Part model, mm, in its own coordinate system. Face numbers are marked on the shaded views. Round coordinates to 2 decimals unless told otherwise and drop trailing zeros. Order: outer loops, then holes, each group sorted by start corner. A loop starts at its lowest first (then second) coordinate and runs counter-clockwise, first axis right, second up. Notation, with made-up numbers: (-7, 9) - (39, 9) arc R22 ccw to (39, 21) - close; hole circle Ø8 at (12, 31). An arc over 180 degrees is marked (long way). Return JSON: item names as keys, results as strings. Group by question number.
Item 1: Probe probe 1 along X at (y, z) = (-1.5, -19) (3 decimals); probe 2 along X at (y, z) = (-0.75, -23) (3 decimals); probe 3 along X at (y, z) = (3, -12.5) (3 decimals). List the from-to ranges inside material, lowest first.
Item 2: Two-plate mould, pull along X, no slides. Class the marked faces 1, 2 and 3: released by +X, released by -X, zero draft, split by the parting line, or undercut.
Item 3: Saw through at D-D on z = -25. List the corners of the cut face in (x, y) (1 decimal).
Item 4: Drop flat-ended pins along their axis: pin 1 (1 mm diameter, centred on x = 0, y = -1, fed in from -Z); pin 2 (3 mm diameter, centred on x = 20.5, z = -15.5, fed in from -Y); pin 3 (1 mm diameter, centred on y = 3, z = -3.5, fed in from -X); pin 4 (4.5 mm diameter, centred on x = 32.5, y = -1, fed in from +Z). Give the stop position or say it passes through.
Item 5: Saw through at B-B on z = -19. List the corners of the cut face in (x, y) (1 decimal).
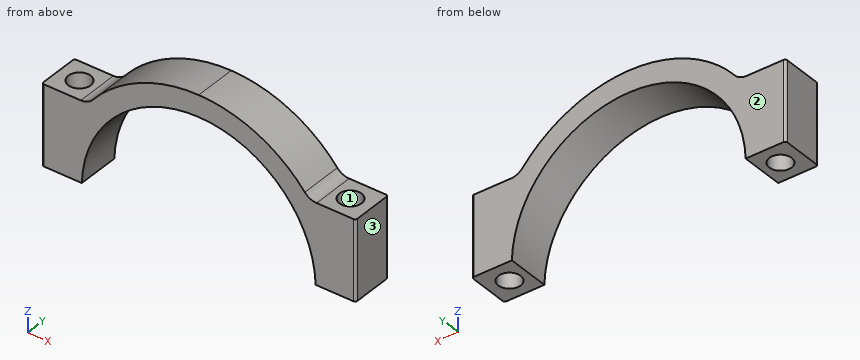
```python
from build123d import *

# Parameters (mm, degrees)
BOSS_EXTRUDE1_DEPTH    = 4.7625
F_10_CLEARANCE_HOLE1_D = 4.9784
CUT_EXTRUDE2_DEPTH     = 48.038415261
FILLET1_R              = 3.429
FILLET2_R              = 0.508


with BuildPart() as part:
    # Sketch1 → Boss-Extrude1 (new, symmetric)
    with BuildSketch(Plane(origin=(0, 0, 0), x_dir=(1, 0, 0), z_dir=(0, 1, 0))):
        with BuildLine():
            Line((-26.023846391, 30.0355), (-34.925, 30.0355))
            Line((-34.925, 30.0355), (-34.925, 0))
            Line((-34.925, 0), (34.925, 0))
            Line((34.925, 0), (34.925, 30.0355))
            Line((34.925, 30.0355), (26.023846391, 30.0355))
            ThreePointArc((26.023846391, 30.0355), (0, 4.7625), (-26.023846391, 30.0355))
        make_face()
    extrude(amount=BOSS_EXTRUDE1_DEPTH, both=True)

    # #10 Clearance Hole1 (through all)
    with Locations(Plane(origin=(0, 0, -30.0355), x_dir=(-1, 0, 0), z_dir=(0, 0, -1))):
        with Locations((-30.1625, 0), (30.1625, 0)):
            Hole(F_10_CLEARANCE_HOLE1_D / 2)

    # Sketch6 → Cut-Extrude2 (cut, through all)
    with BuildSketch(Plane.XZ.offset(4.7625)):
        with BuildLine():
            Line((-24.590246893, -12.2555), (-34.925, -12.2555))
            Line((-34.925, -12.2555), (-34.925, 0))
            Line((-34.925, 0), (0, 0))
            ThreePointArc((0, 0), (-13.737517266, -3.23363551), (-24.590246893, -12.2555))
        make_face()
    cut_extrude2 = extrude(amount=-CUT_EXTRUDE2_DEPTH, mode=Mode.SUBTRACT)

    # Mirror1: Cut-Extrude2 across plane
    add(cut_extrude2.mirror(Plane(origin=(0, 0, 0), x_dir=(0, 0, 1), z_dir=(1, 0, 0))), mode=Mode.SUBTRACT)

    # Fillet1
    fillet1_edges = [part.edges().sort_by_distance(p)[0] for p in [
        (-24.590246893, 0, -12.2555),
        (24.590246893, 0, -12.2555),
    ]]
    fillet(fillet1_edges, radius=FILLET1_R)

    # Fillet2
    fillet2_edges = [part.edges().sort_by_distance(p)[0] for p in [
        (-34.925, 4.7625, -21.1455),
        (34.925, -4.7625, -21.1455),
        (34.925, 4.7625, -21.1455),
        (-34.925, -4.7625, -21.1455),
    ]]
    fillet(fillet2_edges, radius=FILLET2_R)


solid = part.part
```
Filled in:
{
 "1": {"probe 1": "x = -34.925 to -32.149, -28.176 to -23.209, 23.209 to 28.176, 32.149 to 34.925", "probe 2": "x = -34.925 to -32.536, -27.789 to -24.84, 24.84 to 27.789, 32.536 to 34.925", "probe 3": "x = -34.925 to -18.521, 18.521 to 34.925"},
 "2": {"face 1": "undercut", "face 2": "zero draft", "face 3": "released by +X"},
 "3": {"outline": "(-34.9, -4.3) arc R0.5 ccw to (-34.4, -4.8) - (-25.4, -4.8) - (-25.4, 4.8) - (-34.4, 4.8) arc R0.5 ccw to (-34.9, 4.3) - close; (25.4, -4.8) - (34.4, -4.8) arc R0.5 ccw to (34.9, -4.3) - (34.9, 4.3) arc R0.5 ccw to (34.4, 4.8) - (25.4, 4.8) - close; hole circle Ø5 at (-30.2, 0); hole circle Ø5 at (30.2, 0)"},
 "4": {"pin 1": "stops at z = -4.77", "pin 2": "stops at y = -4.76", "pin 3": "stops at x = -15.18", "pin 4": "stops at z = -12.26"},
 "5": {"outline": "(-34.9, -4.3) arc R0.5 ccw to (-34.4, -4.8) - (-23.2, -4.8) - (-23.2, 4.8) - (-34.4, 4.8) arc R0.5 ccw to (-34.9, 4.3) - close; (23.2, -4.8) - (34.4, -4.8) arc R0.5 ccw to (34.9, -4.3) - (34.9, 4.3) arc R0.5 ccw to (34.4, 4.8) - (23.2, 4.8) - close; hole circle Ø5 at (-30.2, 0); hole circle Ø5 at (30.2, 0)"}
}
